Read the model definition and answer for the solid it produces. Units are mm, in the model's axes. A direction names the side the tool comes from. Give positions to 0.01 mm unless a question says otherwise; leave off trailing zeros. Order: outer loops, then holes, each group sorted by start corner. A loop starts at its lowest first (then second) coordinate and runs counter-clockwise, first axis right, second up.
```python
from build123d import *

# Parameters (mm, degrees)
SKETCH2_R           = 0.5
BOSS_EXTRUDE1_DEPTH = 2.5


with BuildPart() as part:
    # Sketch2 → Boss-Extrude1 (new, symmetric)
    with BuildSketch(Plane.XY):
        Polygon((-5, 0), (5, 0), (5, 2), (3, 2), (3, 5), (1, 5), (1, 7), (-1, 7), (-1, 5), (-3, 5), (-3, 2), (-5, 2), align=None)
        with Locations((0, 5)):
            Circle(SKETCH2_R, mode=Mode.SUBTRACT)
        with BuildLine():
            ThreePointArc((-1.75, 1.968911087), (0, 1.5), (1.75, 1.968911087))
            ThreePointArc((1.75, 1.968911087), (1.933012702, 2.651923789), (1.25, 2.834936491))
            ThreePointArc((1.25, 2.834936491), (0, 2.5), (-1.25, 2.834936491))
            ThreePointArc((-1.25, 2.834936491), (-1.933012702, 2.651923789), (-1.75, 1.968911087))
        make_face(mode=Mode.SUBTRACT)
    extrude(amount=BOSS_EXTRUDE1_DEPTH, both=True)


solid = part.part
```
1) A tool of negligible diameter and unlimited length cuts with its end or side. For faces 4 (the face through (4, 2, 0)), 5 (the face through (0, 0, 0)), 6 (the face through (0, 1.5, 0)), 7 (the face through (-3, 4, 0)), from which of +Z, -Z, +X, -X, +Y, -Y can it reach the whole face along a straight path? Write none if from no direction.
Final values:
face 4: +Z, -Z, +X, +Y
face 5: +Z, -Z, +X, -X, -Y
face 6: +Z, -Z
face 7: +Z, -Z, -X, +Y
2) Consider L1, parallel to Y at x = 0, z = -1.1; L2, parallel to Y at x = -0.25, z = -0.6; L3, parallel to Y at x = -4.5, z = -1.85. Determine where each line is inside the solid, lowest interval first.
Final values:
L1: y = 0 to 1.5, 2.5 to 4.5, 5.5 to 7
L2: y = 0 to 1.51, 2.51 to 4.57, 5.43 to 7
L3: y = 0 to 2
3) The part is cut by section D-D on x = -1.5. Determine the outline of the cut face in (y, z).
Final values:
outline: (0, -2.5) - (1.84, -2.5) - (1.84, 2.5) - (0, 2.5) - close; (2.9, -2.5) - (5, -2.5) - (5, 2.5) - (2.9, 2.5) - close
4) The part is cut by section C-C on y = 1.75. Determine the outline of the cut face in (x, z), and give its area (3 significant figures).
Final values:
outline: (-5, -2.5) - (-1.3, -2.5) - (-1.3, 2.5) - (-5, 2.5) - close; (1.3, -2.5) - (5, -2.5) - (5, 2.5) - (1.3, 2.5) - close
area: 37.0 mm2
5) The part is cut by section B-B on x = 0. Determine the outline of the cut face in (y, z).
Final values:
outline: (0, -2.5) - (1.5, -2.5) - (1.5, 2.5) - (0, 2.5) - close; (2.5, -2.5) - (4.5, -2.5) - (4.5, 2.5) - (2.5, 2.5) - close; (5.5, -2.5) - (7, -2.5) - (7, 2.5) - (5.5, 2.5) - close
6) The part is cut by section A-A on z = -0.5. Determine the outline of the cut face in (x, y).
Final values:
outline: (-5, 0) - (5, 0) - (5, 2) - (3, 2) - (3, 5) - (1, 5) - (1, 7) - (-1, 7) - (-1, 5) - (-3, 5) - (-3, 2) - (-5, 2) - close; hole (-1.75, 1.97) arc R3.5 ccw to (1.75, 1.97) arc R0.5 ccw to (1.25, 2.83) arc R2.5 cw to (-1.25, 2.83) arc R0.5 ccw to start; hole circle Ø1 at (0, 5)
7) For a pull along X with two mould halves and no side action, classify faces 1 (the face through (-4, 2, 0)), 2 (the face through (1.94, 2.64, 0.04)), 3 (the face through (1, 6, 0)) as released by +X, released by -X, zero draft, split by the parting line, or undercut.
Final values:
face 1: zero draft
face 2: undercut
face 3: released by +X
8) Given pin 1 (1 mm diameter, centred on x = 2, z = 1, fed in from +Y); pin 2 (1.6 mm diameter, centred on y = 5.5, z = -1, fed in from +X); pin 3 (1 mm diameter, centred on y = 3.5, z = 0.5, fed in from -X), each flat-ended and moving along its own axis, determine where each tip first touches the part or whether it passes through.
Final values:
pin 1: stops at y = 5
pin 2: stops at x = 3
pin 3: stops at x = -3
